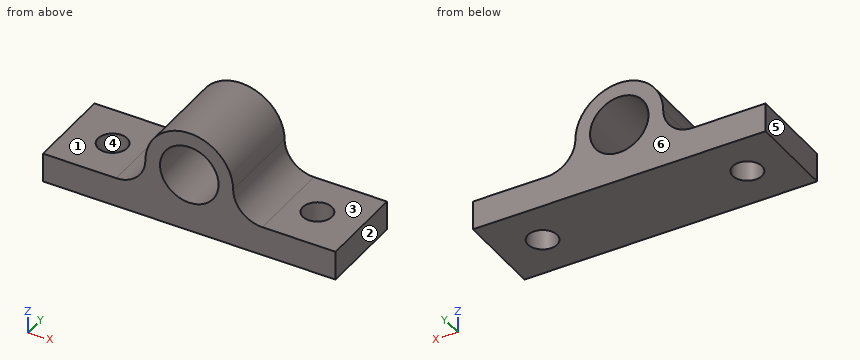
```python
from build123d import *

# Parameters (mm, degrees)
F0_R     = 12.7
F1_DEPTH = 38.1
F2_R     = 6.35
F3_DEPTH = 25.4
F4_R     = 6.35
F5_DEPTH = 25.4


with BuildPart() as f1:
    # F0 (on Front) → F1 (new body)
    with BuildSketch(Plane.XZ):
        with BuildLine():
            Line((-63.5, 0), (0, 0))
            Line((0, 0), (63.5, 0))
            Line((63.5, 0), (63.5, 12.7))
            Line((63.5, 12.7), (31.75, 12.7))
            ThreePointArc((31.75, 12.7), (22.769744, 16.419744), (19.05, 25.4))
            ThreePointArc((19.05, 25.4), (0, 44.45), (-19.05, 25.4))
            ThreePointArc((-19.05, 25.4), (-22.769744, 16.419744), (-31.75, 12.7))
            Line((-31.75, 12.7), (-63.5, 12.7))
            Line((-63.5, 12.7), (-63.5, 0))
        make_face()
        with Locations((0, 25.4)):
            Circle(F0_R, mode=Mode.SUBTRACT)
    extrude(amount=F1_DEPTH)

    # F2 (on face) → F3 (cut)
    with BuildSketch(Plane.XY.offset(12.7)):
        with Locations((44.45, -19.05)):
            Circle(F2_R)
    extrude(amount=-F3_DEPTH, mode=Mode.SUBTRACT)

    # F4 (on face) → F5 (cut)
    with BuildSketch(Plane.XY.offset(12.7)):
        with Locations((-44.45, -19.05)):
            Circle(F4_R)
    extrude(amount=-F5_DEPTH, mode=Mode.SUBTRACT)


solid = f1.part
```
The model under review builds one solid part; all positions refer to its coordinate system, in mm. Face numbers are marked on the shaded views. A direction names the side the tool comes from. Round coordinates to 2 decimals unless told otherwise and drop trailing zeros. Loops run counter-clockwise (first coordinate to the right, second up) from the corner with the lowest first, then second, coordinate; pieces in that order, holes last. Notation, with made-up numbers: (75, 59) - (127, 59) arc R28 ccw to (127, 86) - close; hole circle Ø6 at (89, 59). An arc over 180 degrees is marked (long way). Use a Markdown table: item, result. Add a question column.
Q1. Add section D-D (z = 9). State the section outline as (x, y) points.
Q2. Add section C-C (y = -9.5). State the section outline as (x, z) points, plus the area to 3 significant figures.
Q3. Add section B-B (x = 0). State the section outline as (y, z) points, plus the area to 3 significant figures.
Q4. Machinability: for the marked faces 1, 2 and 3, which of the approach directions +Z, -Z, +X, -X, +Y, -Y give a long, thin tool a straight path to every point of the face, cutting with its end or side? Answer none if there is none.
Q5. The part is to be moulded in two halves that separate along Y. For the marked faces 4, 5 and 6, say which applies: pulls with the +Y half, pulls with the -Y half, needs draft (parallel to the pull), parting line crosses it, or undercut.
Q6. Add section A-A (y = -19.05). State the section outline as (x, z) points.
Q7. Insertion check: pin 1 Ø16 at (x, y) = (-45.5, -27) entering from +Z; pin 2 Ø6 at (y, z) = (-16.5, 32) entering from -X. Each pin has a flat end and moves straight along its axis. Give the tip position at first contact, or say it passes through.
Q8. For probe 1 along X at (y, z) = (-12, 25); probe 2 along Z at (x, y) = (0, -10.5); probe 3 along Z at (x, y) = (-34, -14.5), list the stretches that pass through material, from the lowest coordinate up.
Worked answers:
| question | item | result |
|---|---|---|
| 1 | outline | (-63.5, -38.1) - (63.5, -38.1) - (63.5, 0) - (-63.5, 0) - close; hole circle Ø12.7 at (-44.45, -19.05); hole circle Ø12.7 at (44.45, -19.05) |
| 2 | outline | (-63.5, 0) - (63.5, 0) - (63.5, 12.7) - (31.75, 12.7) arc R12.7 cw to (19.05, 25.4) arc R19.05 ccw to (-19.05, 25.4) arc R12.7 cw to (-31.75, 12.7) - (-63.5, 12.7) - close; hole circle Ø25.4 at (0, 25.4) |
| 2 | area | 2,230 mm² |
| 3 | outline | (-38.1, 0) - (0, 0) - (0, 12.7) - (-38.1, 12.7) - close; (-38.1, 38.1) - (0, 38.1) - (0, 44.45) - (-38.1, 44.45) - close |
| 3 | area | 726 mm² |
| 4 | face 1 | +Z, -X, +Y, -Y |
| 4 | face 2 | +Z, -Z, +X, +Y, -Y |
| 4 | face 3 | +Z, +X, +Y, -Y |
| 5 | face 4 | undercut |
| 5 | face 5 | needs draft |
| 5 | face 6 | pulls with the +Y half |
| 6 | outline | (-63.5, 0) - (-50.8, 0) - (-50.8, 12.7) - (-63.5, 12.7) - close; (-38.1, 0) - (38.1, 0) - (38.1, 12.7) - (31.75, 12.7) arc R12.7 cw to (19.05, 25.4) arc R19.05 ccw to (-19.05, 25.4) arc R12.7 cw to (-31.75, 12.7) - (-38.1, 12.7) - close; (50.8, 0) - (63.5, 0) - (63.5, 12.7) - (50.8, 12.7) - close; hole circle Ø25.4 at (0, 25.4) |
| 7 | pin 1 | z = 12.7 |
| 7 | pin 2 | x = -18.71 |
| 8 | probe 1 | -19.06 to -12.69, 12.69 to 19.06 |
| 8 | probe 2 | 0 to 12.7, 38.1 to 44.45 |
| 8 | probe 3 | 0 to 12.7 |
